The figure shows three views and two pictorial views of one solid part (mm, origin at its lowest corner). Answer the questions. A direction names the side the tool comes from. Coordinates: 2 decimals unless noted, no trailing zeros. Order: outer loops, then holes, each group sorted by start corner. A loop starts at its lowest first (then second) coordinate and runs counter-clockwise, first axis right, second up. Notation, with made-up numbers: (82.5, 5.5) -> (136.5, 5.5) arc R33 cw to (136.5, 33.5) -> close; hole circle Ø3 at (87, -22.75). An arc over 180 degrees is marked (long way). Return JSON: item names as keys, results as strings.
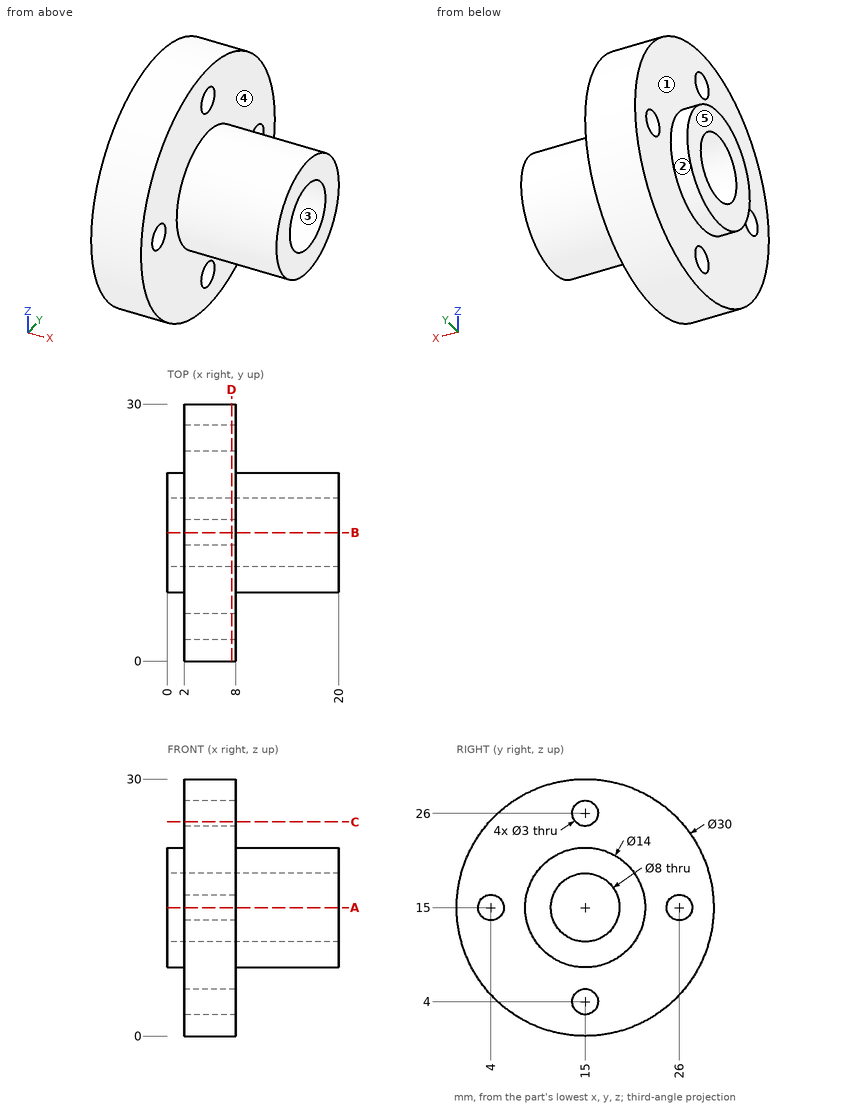
1. The part is cut by section D-D on x = 7.5. Give the vertices of the cut face in (y, z), and give its area (3 significant figures).
Answer block:
{"outline": "circle Ø30 at (15, 15); hole circle Ø3 at (4, 15); hole circle Ø8 at (15, 15); hole circle Ø3 at (15, 4); hole circle Ø3 at (15, 26); hole circle Ø3 at (26, 15)", "area": "628 mm2"}
2. The part is cut by section C-C on z = 25. Give the vertices of the cut face in (x, y).
Answer block:
{"outline": "(2, 3.82) -> (8, 3.82) -> (8, 13.88) -> (2, 13.88) -> close; (2, 16.12) -> (8, 16.12) -> (8, 26.18) -> (2, 26.18) -> close"}
3. Consider line 1 (Y direction, x = 6.1, z = 15); line 2 (Z direction, x = 5.5, y = 15.75); line 3 (Z direction, x = 1.25, y = 15.25). Determine where each line is inside the solid, lowest interval first. Write a range as from..to.
Answer block:
{"line 1": "y = 0..2.5, 5.5..11, 19..24.5, 27.5..30", "line 2": "z = 0.02..2.7, 5.3..11.07, 18.93..24.7, 27.3..29.98", "line 3": "z = 8..11.01, 18.99..22"}
4. Each of these flat-tipped pins is pushed along its axis until it touches: pin 1 Ø2 at (y, z) = (18, 25.5) entering from +X; pin 2 Ø10 at (x, y) = (14, 7.5) entering from +Z; pin 3 Ø3.5 at (y, z) = (15, 26) entering from -X; pin 4 Ø6.5 at (y, z) = (15, 15) entering from +X. Where does it stop, or does it pass through?
Answer block:
{"pin 1": "stops at x = 8", "pin 2": "stops at z = 21.54", "pin 3": "stops at x = 2", "pin 4": "passes through"}
5. The part is cut by section A-A on z = 15. Give the vertices of the cut face in (x, y), and give its area (3 significant figures).
Answer block:
{"outline": "(0, 8) -> (2, 8) -> (2, 5.5) -> (8, 5.5) -> (8, 8) -> (20, 8) -> (20, 11) -> (0, 11) -> close; (0, 19) -> (20, 19) -> (20, 22) -> (8, 22) -> (8, 24.5) -> (2, 24.5) -> (2, 22) -> (0, 22) -> close; (2, 0) -> (8, 0) -> (8, 2.5) -> (2, 2.5) -> close; (2, 27.5) -> (8, 27.5) -> (8, 30) -> (2, 30) -> close", "area": "180 mm2"}
6. Determine the mould class of the marked faces 1, 2 and 3 for opening direction Y: pulls with the +Y half, pulls with the -Y half, needs draft (parallel to the pull), parting line crosses it, or undercut.
Answer block:
{"face 1": "needs draft", "face 2": "parting line crosses it", "face 3": "undercut"}
7. For the marked faces 4 and 5, determine the directions among +Z, -Z, +X, -X, +Y, -Y from which every point of the face is accessible in a straight line to the end or side of a thin tool.
Answer block:
{"face 4": "+X", "face 5": "+Z, -Z, -X, +Y, -Y"}
